Here's how the part is built. I have some questions about the finished solid (model axes, mm). Round coordinates to 2 decimals unless told otherwise and drop trailing zeros. Write each loop counter-clockwise with the first axis right and the second up, starting at its lowest first coordinate (ties: lowest second). Pieces come first, ordered by that corner, then holes. Notation, with made-up numbers: (-26, 46) -> (-21, 46) arc R8 ccw to (-21, 57) -> close; hole circle Ø4 at (-22.75, 19.25). An arc over 180 degrees is marked (long way). Answer as CSV lines item,"result".
from build123d import *

# Parameters (mm, degrees)
FASE1_SIZE = 0.4


with BuildPart() as part:
    # Skizze5 → Rotation1 (revolve)
    with BuildSketch(Plane(origin=(0, 0, 0), x_dir=(0, 0, -1), z_dir=(1, 0, 0)), mode=Mode.PRIVATE) as rotation1_sk:
        Polygon((0, 2.6), (-5.6, 2.6), (-5.6, 3.5), (-0.415050889, 6.740593194), (0, 6.325542305), align=None)
    revolve(rotation1_sk.sketch.rotate(Axis((0, 0, 0), (0, 0, 1)), 90), axis=Axis((0, 0, 0), (0, 0, 1)))

    # Fase1
    fase1_edges = [part.edges().sort_by_distance(p)[0] for p in [
        (2.6, 0, 5.6),
        (2.6, 0, 0),
    ]]
    chamfer(fase1_edges, length=FASE1_SIZE)


solid = part.part
Item 1: Suppose I cut it at A-A, the plane y = 0. List the corners of the cut face in (x, z) for me, then the cut area to 3 significant figures.
Results found:
outline,"(-6.74, 0.42) -> (-6.33, 0) -> (-3, 0) -> (-2.6, 0.4) -> (-2.6, 5.2) -> (-3, 5.6) -> (-3.5, 5.6) -> close; (2.6, 0.4) -> (3, 0) -> (6.33, 0) -> (6.74, 0.42) -> (3.5, 5.6) -> (3, 5.6) -> (2.6, 5.2) -> close"
area,"29.1 mm²"
Item 2: Suppose I cut it at D-D, the plane z = 2.3. List the corners of the cut face in (x, y) for me (1 decimal), then the cut area to 3 significant figures.
Results found:
outline,"circle Ø11.1 at (0, 0); hole circle Ø5.2 at (0, 0)"
area,"76.0 mm²"
Item 3: Will these pins go through, and if not, where does the flat tip stop? pin 1 (3 mm diameter, centred on x = -5, y = -5.5, fed in from -Z); pin 2 (2 mm diameter, centred on y = 4, z = 2.5, fed in from +X); pin 3 (4.5 mm diameter, centred on x = 0, y = 0, fed in from +Z); pin 4 (1.5 mm diameter, centred on x = 5, y = -2, fed in from +Z).
Results found:
pin 1,"stops at z = 0"
pin 2,"stops at x = 4.87"
pin 3,"passes through"
pin 4,"stops at z = 3.78"
Item 4: If we mould it in two halves opening along Z, with no side actions, what happens to faces 1 (the conical face through (0.8, 3.6, 5.3)), 2 (the flat face through (-3, 1, 0)), 3 (the cylindrical face through (0.338, -2.578, 2.834))? For each: pulls with the +Z half, pulls with the -Z half, needs draft (parallel to the pull), parting line crosses it, or undercut.
Results found:
face 1,"pulls with the +Z half"
face 2,"pulls with the -Z half"
face 3,"needs draft"
Item 5: Suppose I cut it at C-C, the plane z = 4.25. List the corners of the cut face in (x, y) for me.
Results found:
outline,"circle Ø8.69 at (0, 0); hole circle Ø5.2 at (0, 0)"
Item 6: I need wall thicknesses on L1, parallel to Y at x = 0, z = 2.15; L2, parallel to Y at x = 0, z = 3.35; L3, parallel to X at y = -2, z = 4.3. Which ranges of each line are inside material? Lowest first, please.
Results found:
L1,"y = -5.66 to -2.6, 2.6 to 5.66"
L2,"y = -4.91 to -2.6, 2.6 to 4.91"
L3,"x = -3.82 to -1.66, 1.66 to 3.82"
